Read the model definition and answer for the solid it produces. Units are mm, in the model's axes. Round coordinates to 2 decimals unless told otherwise and drop trailing zeros. Order: outer loops, then holes, each group sorted by start corner. A loop starts at its lowest first (then second) coordinate and runs counter-clockwise, first axis right, second up.
from build123d import *

# Parameters (mm, degrees)
F0_R     = 203.2
F0_R_2   = 158.75
F1_DEPTH = 38.1
F2_R     = 19.04999
F3_DEPTH = 38.1
F4_SIZE  = 5.08
F5_SIZE  = 5.08


# Not quite as in the source:
# - a fillet or chamfer is up to 0.001 mm smaller than in the source, because OpenCascade refuses the exact size


with BuildPart() as f1:
    # F0 (on Front) → F1 (new body)
    with BuildSketch(Plane.XZ):
        Circle(F0_R)
        Circle(F0_R_2, mode=Mode.SUBTRACT)
    extrude(amount=F1_DEPTH)

    # F2 (radius 19.05 in the source; OpenCascade refuses exactly that, so slightly less here)
    f2_edges = [f1.edges().sort_by_distance(p)[0] for p in [
        (-203.2, -38.1, 0),
        (-203.2, 0, 0),
    ]]
    fillet(f2_edges, radius=F2_R)

    # F3 (add): a face of the model
    f3_faces = [f1.faces().sort_by_distance(p)[0] for p in [
        (-178.9414611669, 0, 0),
    ]]
    extrude(f3_faces, amount=-F3_DEPTH)

    # F4
    f4_edges = [f1.edges().sort_by_distance(p)[0] for p in [
        (-158.75, -38.1, 0),
    ]]
    chamfer(f4_edges, length=F4_SIZE)

    # F5
    f5_edges = [f1.edges().sort_by_distance(p)[0] for p in [
        (-158.75, 0, 0),
    ]]
    chamfer(f5_edges, length=F5_SIZE)


solid = f1.part
Q1. Flat-ended cylindrical pins translate along their axes: pin 1 (3 mm diameter, centred on y = -17, z = -118.5, fed in from +X); pin 2 (8 mm diameter, centred on y = -32, z = -86.5, fed in from -X); pin 3 (4 mm diameter, centred on y = -32.5, z = -156.5, fed in from +X). Find the tip coordinate at first contact, or state that the pin passes through.
Outcome:
pin 1: stops at x = 166.02
pin 2: stops at x = -182.03
pin 3: stops at x = 124.56
Q2. For a pull along X with two mould halves and no side action, classify faces 1 (the face through (151.42, -18.85, 47.68)), 2 (the face through (-124, -38.1, -108)) as released by +X, released by -X, zero draft, split by the parting line, or undercut.
Outcome:
face 1: undercut
face 2: zero draft
Q3. Straight lines are drawn through the part: probe 1 along Z at (x, y) = (0, -20.5); probe 2 along Z at (x, y) = (0, -15); probe 3 along X at (y, z) = (-15, -8.5). For each, find the intervals that lie inside material, in ascending order.
Outcome:
probe 1: z = -203.14 to -158.75, 158.75 to 203.14
probe 2: z = -202.76 to -158.75, 158.75 to 202.76
probe 3: x = -202.59 to -158.52, 158.52 to 202.59
Q4. A cutting plane is placed at C-C, the plane y = -14. Give the vertices of the cut face in (x, z), plus the area to 3 significant figures.
Outcome:
outline: circle Ø405.04 at (0, 0); hole circle Ø317.5 at (0, 0)
area: 49,700 mm2
